```python
from build123d import *

# Parameters (mm, degrees)
BOSS_EXTRUDE1_DEPTH = 5
SKETCH3_W           = 17.5
SKETCH3_H           = 12
SKETCH3_W_2         = 5.5
SKETCH3_R           = 1.5
CUT_EXTRUDE1_DEPTH  = 81.777472107
SKETCH5_R           = 3
CUT_EXTRUDE2_DEPTH  = 2
CUT_EXTRUDE3_DEPTH  = 2
SKETCH8_R           = 1.5
CUT_EXTRUDE4_DEPTH  = 81.678373806


with BuildPart() as part:
    # Sketch1 → Boss-Extrude1 (new body)
    with BuildSketch(Plane(origin=(0, 0, 0), x_dir=(1, 0, 0), z_dir=(0, 1, 0))):
        with BuildLine():
            Line((-40, 10), (40, 10))
            ThreePointArc((40, 10), (50, 0), (40, -10))
            Line((40, -10), (-40, -10))
            Line((-40, -10), (-70, -10))
            ThreePointArc((-70, -10), (-80, 0), (-70, 10))
            Line((-70, 10), (-40, 10))
        make_face()
    extrude(amount=BOSS_EXTRUDE1_DEPTH)

    # Sketch3 → Cut-Extrude1 (cut, through all)
    with BuildSketch(Plane(origin=(0, 5, 0), x_dir=(1, 0, 0), z_dir=(0, 1, 0))):
        with Locations((31.25, 0)):
            Rectangle(SKETCH3_W, SKETCH3_H)
        with Locations((42.75, 0)):
            Rectangle(SKETCH3_W_2, SKETCH3_H)
        with Locations(Location((20.5, 0, 0), (0, 0, 270))):
            Circle(SKETCH3_R)
        with Locations(Location((47.5, 0, 0), (0, 0, 270))):
            Circle(SKETCH3_R)
    extrude(amount=-CUT_EXTRUDE1_DEPTH, mode=Mode.SUBTRACT)

    # Sketch5 → Cut-Extrude2 (cut)
    with BuildSketch(Plane(origin=(0, 5, 0), x_dir=(1, 0, 0), z_dir=(0, 1, 0))):
        with Locations(Location((-70, 0, 0), (0, 0, 270))):
            Circle(SKETCH5_R)
    extrude(amount=-CUT_EXTRUDE2_DEPTH, mode=Mode.SUBTRACT)

    # Sketch6 → Cut-Extrude3 (cut)
    with BuildSketch(Plane.XZ):
        with BuildLine():
            Line((-71.152960707, 6.396927513), (-78.631797828, 5.04896685))
            ThreePointArc((-78.631797828, 5.04896685), (-79.999926685, 0.038292326), (-78.670211746, -4.982712945))
            Line((-78.670211746, -4.982712945), (-70, -6.5))
            Line((-70, -6.5), (-50, -3))
            ThreePointArc((-50, -3), (-47, 0), (-50, 3))
            Line((-50, 3), (-68.847039198, 6.396927496))
            ThreePointArc((-68.847039198, 6.396927496), (-69.999999952, 6.5), (-71.152960707, 6.396927513))
        make_face()
    extrude(amount=-CUT_EXTRUDE3_DEPTH, mode=Mode.SUBTRACT)

    # Sketch8 → Cut-Extrude4 (cut, through all)
    with BuildSketch(Plane(origin=(0, 3, 0), x_dir=(1, 0, 0), z_dir=(0, 1, 0))):
        with Locations(Location((-70, 0, 0), (0, 0, 270))):
            Circle(SKETCH8_R)
    extrude(amount=-CUT_EXTRUDE4_DEPTH, mode=Mode.SUBTRACT)


solid = part.part
```
Geometry: final body of the model. Coordinates: model frame, mm. A direction names the side the tool comes from. Round coordinates to 2 decimals unless told otherwise and drop trailing zeros. Loops run counter-clockwise (first coordinate to the right, second up) from the corner with the lowest first, then second, coordinate; pieces in that order, holes last. Notation, with made-up numbers: (-19.75, 79) -> (1.25, 79) arc R20 cw to (1.25, 102) -> close; hole circle Ø4 at (78, -20). An arc over 180 degrees is marked (long way). Use one line per item in the form item = value.
Item 1: Cut plane C-C on x = 20.5. Output: boundary loops of the cut face in (y, z).
Evaluation:
outline = (0, -10) -> (5, -10) -> (5, -1.5) -> (0, -1.5) -> close; (0, 1.5) -> (5, 1.5) -> (5, 10) -> (0, 10) -> close
Item 2: Cut plane D-D on x = 47.5. Output: boundary loops of the cut face in (y, z).
Evaluation:
outline = (0, -6.61) -> (5, -6.61) -> (5, -1.5) -> (0, -1.5) -> close; (0, 1.5) -> (5, 1.5) -> (5, 6.61) -> (0, 6.61) -> close
Item 3: Material intervals for probe 1 along X at (y, z) = (2.4, 0); probe 2 along X at (y, z) = (4.15, 0); probe 3 along Z at (x, y) = (35, 1.65), sorted ascending.
Evaluation:
probe_1 = -80 to -71.5, -68.5 to 19, 22 to 22.5, 45.5 to 46, 49 to 50
probe_2 = -80 to -73, -67 to 19, 22 to 22.5, 45.5 to 46, 49 to 50
probe_3 = -10 to -6, 6 to 10
Item 4: Contact query for flat-ended pins moving along their axis: pin 1 Ø1.5 at (y, z) = (3.5, -2) entering from +X; pin 2 Ø1 at (x, z) = (-59, 2) entering from -Y; pin 3 Ø3.5 at (x, z) = (-70, 0) entering from +Y; pin 4 Ø6.5 at (x, z) = (-61, -2) entering from -Y. Output: stop coordinate, or through.
Evaluation:
pin_1 = 49.92
pin_2 = 2
pin_3 = 3
pin_4 = 0
Item 5: Draft query along X for faces 1 (the cylindrical face through (50, 2, 0)), 2 (the flat face through (-16, 2, -10)), 3 (the flat face through (34, 3, 6)). Return one class per face: released by +X, released by -X, zero draft, split by the parting line, or undercut.
Evaluation:
face_1 = released by +X
face_2 = zero draft
face_3 = undercut
Item 6: Access query for faces 4 (the flat face through (-14, 5, 0)), 5 (the cylindrical face through (-47, 1, 0)), 6 (the cylindrical face through (-72.93, 4.01, -0.65)), 7 (the flat face through (-74.4, 0.99, -5.73)), 8 (the flat face through (22.5, 3, 0)). Directions: +Z, -Z, +X, -X, +Y, -Y. A direction counts if a zero-diameter tool reaches every point of the face in a straight line with its end or side. Return the directions, or none.
Evaluation:
face_4 = +Z, -Z, +X, -X, +Y
face_5 = -X, -Y
face_6 = +Y
face_7 = -Y
face_8 = +Y, -Y
Item 7: Cut plane A-A on z = 0. Output: boundary loops of the cut face in (x, y), then the cut area to 3 significant figures.
Evaluation:
outline = (-80, 2) -> (-71.5, 2) -> (-71.5, 3) -> (-73, 3) -> (-73, 5) -> (-80, 5) -> close; (-68.5, 2) -> (-47, 2) -> (-47, 0) -> (19, 0) -> (19, 5) -> (-67, 5) -> (-67, 3) -> (-68.5, 3) -> close; (22, 0) -> (22.5, 0) -> (22.5, 5) -> (22, 5) -> close; (45.5, 0) -> (46, 0) -> (46, 5) -> (45.5, 5) -> close; (49, 0) -> (50, 0) -> (50, 5) -> (49, 5) -> close
area = 424 mm2
Item 8: Cut plane B-B on y = 4.15. Output: boundary loops of the cut face in (x, z), then the cut area to 3 significant figures.
Evaluation:
outline = (-70, -10) -> (40, -10) arc R10 ccw to (40, 10) -> (-70, 10) arc R10 ccw to start; hole circle Ø6 at (-70, 0); hole circle Ø3 at (20.5, 0); hole (22.5, -6) -> (45.5, -6) -> (45.5, 6) -> (22.5, 6) -> close; hole circle Ø3 at (47.5, 0)
area = 2,200 mm2
